Design review of the part built by this model. Coordinates are the model's own, in mm. A direction names the side the tool comes from. Round coordinates to 2 decimals unless told otherwise and drop trailing zeros. Write each loop counter-clockwise with the first axis right and the second up, starting at its lowest first coordinate (ties: lowest second). Pieces come first, ordered by that corner, then holes. Notation, with made-up numbers: (-37.75, 58.25) -> (-2.75, 58.25) arc R29 cw to (-2.75, 90.25) -> close; hole circle Ø6 at (-4.5, -10.5). An arc over 180 degrees is marked (long way). Write item = value, one per line. Start each with the question number.
Item 1: Add section B-B, the plane x = 13.5. State the section outline as (y, z) points.
Item 2: Add section C-C, the plane z = 12.5. State the section outline as (x, y) points, then the cut area to 3 significant figures.
Item 3: Add section A-A, the plane x = 0. State the section outline as (y, z) points, then the cut area to 3 significant figures.
Item 4: Add section D-D, the plane y = -7.75. State the section outline as (x, z) points, then the cut area to 3 significant figures.
Item 5: For pin 1 Ø10 at (x, y) = (-1.5, -6) entering from +Z; pin 2 Ø4 at (x, y) = (0, 0) entering from -Z; pin 3 Ø10 at (x, y) = (19, 0.5) entering from +Z; pin 4 Ø8 at (x, z) = (19.5, 9) entering from -Y, all flat-tipped, find the tip position at first contact; note any pin that passes through.
Item 6: Machinability: for faces 1 (the flat face through (0, 4.1, 1.2)), 2 (the flat face through (19, -2, 6)), 3 (the flat face through (11.4, 4.8, 2.2)), which of the approach directions +Z, -Z, +X, -X, +Y, -Y give a long, thin tool a straight path to every point of the face, cutting with its end or side? Answer none if there is none.
Item 7: To check wall thickness, follow L1, parallel to Y at x = 0, z = 0.75; L2, parallel to Y at x = 22, z = 1.5; L3, parallel to Z at x = 6.5, y = 4. State the ranges of each line that lie inside material, in increasing order.
Item 8: Mouldability with a two-part tool opening along Y and no side actions: class faces 4 (the flat face through (11.472, -4.673, 2.157)), 5 (the cylindrical face through (3.233, -1.341, 0.597)), 6 (the flat face through (19, 2, 6)) as released by +Y, released by -Y, zero draft, split by the parting line, or undercut.
from build123d import *

# Parameters (mm, degrees)
F0_W        = 18
F0_H        = 18
F0_R        = 3.5
F1_DEPTH    = 1.2
F3_DEPTH    = 15
F4_T4_DEPTH = 90.007123663
F5_SIZE     = 0.4
F6_T1_DEPTH = 24.6


# Not quite as in the source:
# - a fillet or chamfer that OpenCascade refuses, or shapes differently, is made with other operations: its cross-section is extruded or revolved along the edge and cut away or added


with BuildPart() as f1:
    # F0 (on Top) → F1 (new body)
    with BuildSketch(Plane.XY):
        Rectangle(F0_W, F0_H)
        Circle(F0_R, mode=Mode.SUBTRACT)
    extrude(amount=F1_DEPTH)

    # F2 (on face) → F3 (join)
    with BuildSketch(Plane(origin=(0, 0, 0), x_dir=(1, 0, 0), z_dir=(0, 0, -1))):
        Polygon((9, 0), (9, -9), (13, -2), (25, -2), (25, 0), align=None)
        Polygon((9, 9), (9, 0), (25, 0), (25, 2), (13, 2), align=None)
    extrude(amount=-F3_DEPTH)

    # F4: chamfer of 14 on 1 edges, made by hand


with BuildPart() as f4_tool2:
    # F4_s3 → F4_t4 (new body)
    with BuildSketch(Plane.XZ.offset(45.0035618315)):
        Polygon((9, 1), (23, 15), (9, 15), align=None)
    extrude(amount=-F4_T4_DEPTH)

    split(bisect_by=Plane.XY.offset(1.2), keep=Keep.TOP)


with BuildPart() as f1_1:
    add(f1.part)

    # F4_t1: cut F4_tool2
    add(f4_tool2.part, mode=Mode.SUBTRACT)

    # F5
    f5_edges = [f1_1.edges().sort_by_distance(p)[0] for p in [
        (0, -9, 0),
        (11, -5.5, 0),
        (19, -2, 0),
        (25, 0, 0),
        (19, 2, 0),
        (11, 5.5, 0),
        (0, 9, 0),
        (-9, 0, 0),
        (-3.5, 0, 0),
        (-3.5, 0, 1.2),
    ]]
    chamfer(f5_edges, length=F5_SIZE)

    # F6: fillet of radius 2 on 2 edges, made by hand

    # F6_s2 → F6_t1 (cut)
    with BuildSketch(Plane.XY.offset(-4.6)):
        with BuildLine():
            ThreePointArc((23, -2), (24.4142135624, -1.4142135624), (25, 0))
            Line((25, 0), (25, -2))
            Line((25, -2), (23, -2))
        make_face()
        with BuildLine():
            ThreePointArc((23, 2), (24.4142135624, 1.4142135624), (25, 0))
            Line((25, 0), (25, 2))
            Line((25, 2), (23, 2))
        make_face()
    extrude(amount=F6_T1_DEPTH, mode=Mode.SUBTRACT)


solid = f1_1.part
Result set:
q1.outline = (-2, 0.4) -> (-1.6, 0) -> (1.6, 0) -> (2, 0.4) -> (2, 5.5) -> (-2, 5.5) -> close
q2.outline = (20.5, -2) -> (23, -2) arc R2 ccw to (23, 2) -> (20.5, 2) -> close
q2.area = 16.3 mm²
q3.outline = (-9, 0.4) -> (-8.6, 0) -> (-3.9, 0) -> (-3.5, 0.4) -> (-3.5, 0.8) -> (-3.9, 1.2) -> (-9, 1.2) -> close; (3.5, 0.4) -> (3.9, 0) -> (8.6, 0) -> (9, 0.4) -> (9, 1.2) -> (3.9, 1.2) -> (3.5, 0.8) -> close
q3.area = 12.7 mm²
q4.outline = (-9, 0.4) -> (-8.6, 0) -> (9.25, 0) -> (9.71, 0.4) -> (9.71, 1.71) -> (9.2, 1.2) -> (-9, 1.2) -> close
q4.area = 22.4 mm²
q5.pin_1 = 1.2
q5.pin_2 = through
q5.pin_3 = 15
q5.pin_4 = -2
q6.face_1 = +Z, -X, +Y, -Y
q6.face_2 = +Z, -Z, +X, -Y
q6.face_3 = +Z, -Z, +X, +Y
q7.L1 = -9 to -3.5, 3.5 to 9
q7.L2 = -2 to 2
q7.L3 = 0 to 1.2
q8.face_4 = released by -Y
q8.face_5 = undercut
q8.face_6 = released by +Y
